Geometry check sheet. Reference: the model listing, model coordinates, mm. Round coordinates to 2 decimals unless told otherwise and drop trailing zeros. Loops run counter-clockwise (first coordinate to the right, second up) from the corner with the lowest first, then second, coordinate; pieces in that order, holes last. Notation, with made-up numbers: M 40.5,-6 L 90.5,-6 A12 cw 90.5,6 Z; hole C 14,66.25 d11. An arc over 180 degrees is marked long. Use one line per item in the form item = value. Start each with the question number.
1. Cross-section at B-B (y = 3). Record the boundary of the cut face in (x, z), then the cut area to 3 significant figures.
2. Material ranges on line 1 (Y direction, x = -75, z = 2.5); line 2 (Y direction, x = -3.5, z = 4.75), recorded low to high.
3. Cross-section at A-A (x = -3). Record the boundary of the cut face in (y, z), then the cut area to 3 significant figures.
4. Draft check along Y on faces 1 (the cylindrical face through (-77.4, 0.57, 4.93)), 2 (the cylindrical face through (-2.26, 40.58, 4.93)), 3 (the flat face through (-40, 45, 5)), 4 (the cylindrical face through (-3.35, 1.44, 4.93)). Enter one of: pulls with the +Y half, pulls with the -Y half, needs draft (parallel to the pull), parting line crosses it, or undercut.
```python
from build123d import *

# Parameters (mm, degrees)
SKETCH1_R           = 1.6
BOSS_EXTRUDE2_DEPTH = 10


with BuildPart() as part:
    # Sketch1 → Boss-Extrude2 (new body)
    with BuildSketch(Plane.XY):
        with BuildLine():
            Line((-78, 42), (-78, 43))
            ThreePointArc((-78, 43), (-77.414213562, 44.414213562), (-76, 45))
            Line((-76, 45), (-75, 45))
            Line((-75, 45), (-3, 45))
            Line((-3, 45), (-2, 45))
            ThreePointArc((-2, 45), (-0.585786438, 44.414213562), (0, 43))
            Line((0, 43), (0, 42))
            Line((0, 42), (0, 3))
            Line((0, 3), (0, 2))
            ThreePointArc((0, 2), (-0.585786438, 0.585786438), (-2, 0))
            Line((-2, 0), (-3, 0))
            Line((-3, 0), (-75, 0))
            Line((-75, 0), (-76, 0))
            ThreePointArc((-76, 0), (-77.414213562, 0.585786438), (-78, 2))
            Line((-78, 2), (-78, 3))
            Line((-78, 3), (-78, 42))
        make_face()
        with Locations((-75, 3)):
            Circle(SKETCH1_R, mode=Mode.SUBTRACT)
        with Locations((-3, 3)):
            Circle(SKETCH1_R, mode=Mode.SUBTRACT)
        with Locations((-3, 42)):
            Circle(SKETCH1_R, mode=Mode.SUBTRACT)
        with Locations((-75, 42)):
            Circle(SKETCH1_R, mode=Mode.SUBTRACT)
    extrude(amount=BOSS_EXTRUDE2_DEPTH)


solid = part.part
```
Reported:
q1.outline = M -78,0 L -76.6,0 L -76.6,10 L -78,10 Z; M -73.4,0 L -4.6,0 L -4.6,10 L -73.4,10 Z; M -1.4,0 L 0,0 L 0,10 L -1.4,10 Z
q1.area = 716 mm²
q2.line_1 = 0 to 1.4, 4.6 to 40.4, 43.6 to 45
q2.line_2 = 0 to 1.48, 4.52 to 40.48, 43.52 to 45
q3.outline = M 0,0 L 1.4,0 L 1.4,10 L 0,10 Z; M 4.6,0 L 40.4,0 L 40.4,10 L 4.6,10 Z; M 43.6,0 L 45,0 L 45,10 L 43.6,10 Z
q3.area = 386 mm²
q4.face_1 = pulls with the -Y half
q4.face_2 = undercut
q4.face_3 = pulls with the +Y half
q4.face_4 = undercut
